Read the model definition and answer for the solid it produces. Units are mm, in the model's axes. A direction names the side the tool comes from. Give positions to 0.01 mm unless a question says otherwise; leave off trailing zeros. Loops run counter-clockwise (first coordinate to the right, second up) from the corner with the lowest first, then second, coordinate; pieces in that order, holes last. Notation, with made-up numbers: (-39.75, 36) - (-30.75, 36) arc R8 ccw to (-30.75, 44) - close; hole circle Ø7 at (2, -7). An arc over 180 degrees is marked (long way). Put each result on its own line as item: value. Start each with the question number.
1. A cutting plane is placed at A-A, the plane z = 2.75. Determine the outline of the cut face in (x, y).
2. For faces 4 (the flat face through (-24.93, 12.605, 12.325)), 5 (the flat face through (-15, 6, 25)), 6 (the flat face through (-10, 14, 23)), 7 (the flat face through (-15, 15, 12)), 8 (the flat face through (-15, 10, 0)), determine the directions among +Z, -Z, +X, -X, +Y, -Y from which every point of the face is accessible in a straight line to the end or side of a thin tool.
3. Given pin 1 Ø1.5 at (x, y) = (-25.5, 15) entering from +Z; pin 2 Ø2 at (x, z) = (-13, 13.5) entering from +Y, each flat-ended and moving along its own axis, determine where each tip first touches the part or whether it passes through.
4. Consider L1, parallel to Y at x = -14.5, z = 21.5; L2, parallel to X at y = 10, z = 22.25; L3, parallel to X at y = 16, z = 9.25. Determine where each line is inside the solid, lowest interval first. Write a range as from..to.
5. A cutting plane is placed at B-B, the plane y = 18.5. Determine the outline of the cut face in (x, z).
6. A cutting plane is placed at D-D, the plane z = 9.25. Determine the outline of the cut face in (x, y).
7. A cutting plane is placed at C-C, the plane x = -6. Determine the outline of the cut face in (y, z), plus the area to 4 significant figures.
8. For a pull along X with two mould halves and no side action, classify faces 1 (the flat face through (0, 10, 10)), 2 (the flat face through (-20, 16, 2)), 3 (the flat face through (-15, 0, 12)) as released by +X, released by -X, zero draft, split by the parting line, or undercut.
```python
from build123d import *

# Parameters (mm, degrees)
BOSS_EXTRUDE1_DEPTH = 25
BOSS_EXTRUDE2_DEPTH = 10
BOSS_EXTRUDE3_DEPTH = 10


with BuildPart() as part:
    # Sketch1 → Boss-Extrude1 (new body)
    with BuildSketch(Plane.XY):
        Polygon((-30, 5), (-20, 5), (-20, 15), (-10, 15), (-10, 10), (0, 10), (0, 0), (-30, 0), align=None)
    extrude(amount=BOSS_EXTRUDE1_DEPTH)

    # Sketch2 → Boss-Extrude2 (add)
    with BuildSketch(Plane(origin=(-10, 0, 0), x_dir=(0, 0, -1), z_dir=(1, 0, 0))):
        Polygon((-25, 10), (0, 10), (0, 25), align=None)
    extrude(amount=BOSS_EXTRUDE2_DEPTH)

    # Sketch3 → Boss-Extrude3 (add)
    with BuildSketch(Plane.ZY.offset(20)):
        Polygon((0, 5), (0, 20), (25, 5), align=None)
    extrude(amount=BOSS_EXTRUDE3_DEPTH)


solid = part.part
```
Return value:
1. outline: (-30, 0) - (0, 0) - (0, 23.35) - (-10, 23.35) - (-10, 15) - (-20, 15) - (-20, 18.35) - (-30, 18.35) - close
2. face 4: +Z, -X, +Y
2. face 5: +Z, +X, -X, +Y, -Y
2. face 6: +Z, +X, +Y
2. face 7: +Z, -Z, +Y
2. face 8: -Z, +X, -X, +Y, -Y
3. pin 1: stops at z = 9.58
3. pin 2: stops at y = 15
4. L1: y = 0..15
4. L2: x = -20..0
4. L3: x = -10..0
5. outline: (-30, 0) - (-20, 0) - (-20, 2.5) - (-30, 2.5) - close; (-10, 0) - (0, 0) - (0, 10.83) - (-10, 10.83) - close
6. outline: (-30, 0) - (0, 0) - (0, 19.45) - (-10, 19.45) - (-10, 15) - (-20, 15) - (-20, 14.45) - (-30, 14.45) - close
7. outline: (0, 0) - (25, 0) - (10, 25) - (0, 25) - close
7. area: 437.5 mm2
8. face 1: released by +X
8. face 2: undercut
8. face 3: zero draft
